Design review of the part built by this model. Coordinates are the model's own, in mm. Coordinates: 2 decimals unless noted, no trailing zeros. Loops run counter-clockwise (first coordinate to the right, second up) from the corner with the lowest first, then second, coordinate; pieces in that order, holes last. Notation, with made-up numbers: M -4.75,-2.5 L 18.25,-2.5 A25 cw 18.25,16.5 Z; hole C -6,78 d11. An arc over 180 degrees is marked long. Write item = value, one per line. Start each with the question number.
Solid Edge part; units mm, degrees
sketch "Sketch1" plane through (0, 0, 0) normal (0, 0, 1) x (1, 0, 0)
  line L0 (0, 123.5) -> (0, 6.5)
  line L1 (13, 6.5) -> (13, 123.5)
  arc A0 (13, 6.5) -> (0, 6.5) centre (6.5, 6.5) cw
  arc A1 (0, 123.5) -> (13, 123.5) centre (6.5, 123.5) cw
extrude "Protrusion1" add sketch "Sketch1" along normal blind 6.5
sketch "Sketch2" plane through (6.5, 0, 0) normal (1, 0, 0) x (0, 1, 0)
  line L0 (3.5, 0) -> (3.5, 1)
  line L1 (3.5, 1) -> (2.6811, 3.25)
  line L2 (3.5, 5.5) -> (2.6811, 3.25)
  line L3 (3.5, 6.5) -> (3.5, 5.5)
  line L4 (6.5, 6.5) -> (3.5, 6.5)
  line L5 (6.5, 6.5) -> (6.5, 0)
  line L6 (3.5, 0) -> (6.5, 0)
revolve "RevolvedCutout1" cut sketch "Sketch2" angle 360 about axis through (6.5, 6.5, 6.5) along (0, 0, -1)
chamfer "Chaflán_2" distance 0.75 angle 45 2 edges at (9.5, 6.5, 6.5) (9.5, 6.5, 0)
pattern_linear "Pattern1" count 10 spacing 13 along (0, 1, 0) of "RevolvedCutout1", "Chaflán_2"
chamfer "Chaflán_37" distance 1.5 angle 45 8 edges at (0, 65, 0) (6.5, 130, 0) (13, 65, 0) (6.5, 0, 0) (0, 65, 6.5) (6.5, 130, 6.5) (13, 65, 6.5) (6.5, 0, 6.5)
(1) To check wall thickness, follow L1, parallel to X at y = 57.5, z = 3.25; L2, parallel to X at y = 19.5, z = 0.9; L3, parallel to Y at x = 10.25, z = 5.5. State the ranges of each line that lie inside material, in increasing order.
(2) Take a section at B-B (x = 5.25). Give the number of separate pieces and of enclosed holes in the cut face, plus the area to 3 significant figures.
(3) Insertion check: pin 1 (5.5 mm diameter, centred on x = 6.5, y = 110.5, fed in from +Z); pin 2 (7 mm diameter, centred on x = 6.5, y = 58.5, fed in from -Z); pin 3 (2 mm diameter, centred on x = 8.5, y = 109.5, fed in from -Z). Each pin has a flat end and moves straight along its axis. Give the tip position at first contact, or say it passes through.
(4) Take a section at A-A (y = 84.5). State the section outline as (x, z) points.
Results list:
q1.L1 = 0 to 2.81, 10.19 to 13
q1.L2 = 0.6 to 3.5, 9.5 to 12.4
q1.L3 = 1.82 to 128.18
q2.separate_pieces = 11
q2.enclosed_holes = 0
q2.area = 432 mm^2
q3.pin_1 = through
q3.pin_2 = 0.25
q3.pin_3 = 0.51
q4.outline = M 0,1.5 L 1.5,0 L 2.75,0 L 3.5,0.75 L 3.5,1 L 2.68,3.25 L 3.5,5.5 L 3.5,5.75 L 2.75,6.5 L 1.5,6.5 L 0,5 Z; M 9.5,0.75 L 10.25,0 L 11.5,0 L 13,1.5 L 13,5 L 11.5,6.5 L 10.25,6.5 L 9.5,5.75 L 9.5,5.5 L 10.32,3.25 L 9.5,1 Z
